Verification items for the finished model (mm, model axes). A direction names the side the tool comes from. Coordinates: 2 decimals unless noted, no trailing zeros. Order: outer loops, then holes, each group sorted by start corner. A loop starts at its lowest first (then second) coordinate and runs counter-clockwise, first axis right, second up.
Q1. Depth check by flat-ended pin: P1, Ø3, axis at x = 2.5, z = 6.5, coming from the +Y side; P2, Ø2, axis at x = 24, y = 18.5, coming from the +Z side; P3, Ø3, axis at x = 29.5, z = 4, coming from the -Y side; P4, Ø1.8, axis at y = 10.5, z = 4.5, coming from the +X side. Enter the tip coordinate at first touch or a pass-through.
Q2. Cross-section at C-C, the plane z = 6.5. Record the boundary of the cut face in (x, y), and give its area (3 significant figures).
Q3. Thickness scan on line 1 (Y direction, x = 36.2, z = 1.5); line 2 (X direction, y = 12.25, z = 6.75); line 3 (X direction, y = 12, z = 1.5). Record the ranges inside material, lowest first.
Q4. Draft check along X on faces 1 (the cylindrical face through (34.7, 13.06, 1.01)), 2 (the flat face through (40, 8, 1)), 3 (the flat face through (27.119, 17.922, 6.028)), 4 (the flat face through (28, 13, 8)). Enter one of: pulls with the +X half, pulls with the -X half, needs draft (parallel to the pull), parting line crosses it, or undercut.
Q5. Cross-section at B-B, the plane y = 15. Record the boundary of the cut face in (x, z).
Q6. Set-up check for faces 5 (the flat face through (33.2, 13, 5)), 6 (the flat face through (0, 8, 4)), 7 (the flat face through (5, 14.5, 5)), 8 (the flat face through (10, 8, 5)): record each of +Z, -Z, +X, -X, +Y, -Y from which the full face is reachable in a straight line by a thin tool's end or side.
Q7. Cross-section at D-D, the plane x = 6. Record the boundary of the cut face in (y, z), and give its area (3 significant figures).
Q8. Cross-section at A-A, the plane x = 36.2. Record the boundary of the cut face in (y, z).
from build123d import *

# Parameters (mm, degrees)
F0_W     = 40
F0_H     = 16
F1_DEPTH = 2
F2_W     = 10
F2_H     = 13
F2_W_2   = 13
F2_H_2   = 6
F3_DEPTH = 6
F4_R     = 1.5
F5_DEPTH = 25
F7_DEPTH = 4


with BuildPart() as f1:
    # F0 (on Top) → F1 (new body)
    with BuildSketch(Plane.XY):
        with Locations((20, 8)):
            Rectangle(F0_W, F0_H)
    extrude(amount=F1_DEPTH)

    # F2 (on face) → F3 (join)
    with BuildSketch(Plane.XY.offset(2)):
        with Locations((5, 8)):
            Rectangle(F2_W, F2_H)
        with Locations((26.7, 13)):
            Rectangle(F2_W_2, F2_H_2)
    extrude(amount=F3_DEPTH)

    # F4 (on face) → F5 (cut)
    with BuildSketch(Plane.XY.offset(2)):
        with Locations((17.2, 12.58387)):
            Circle(F4_R)
        with Locations((36.2, 12.996209)):
            Circle(F4_R)
    extrude(amount=-F5_DEPTH, mode=Mode.SUBTRACT)

    # F6 (on face) → F7 (join)
    with BuildSketch(Plane.XY.offset(8)):
        with BuildLine():
            Line((33.196565, 19.791735), (20.869566, 16))
            Line((20.869566, 16), (21.372473, 16))
            Line((21.372473, 16), (33.448326, 19.669136))
            ThreePointArc((33.448326, 19.669136), (34.091376, 20.578656), (34.9574, 19.878127))
            Line((34.9574, 19.878127), (35.180375, 19.999125))
            ThreePointArc((35.180375, 19.999125), (34.092116, 20.817116), (33.196565, 19.791735))
        make_face()
    extrude(amount=-F7_DEPTH)


solid = f1.part
Check values:
1. P1: stops at y = 14.5
1. P2: passes through
1. P3: stops at y = 10
1. P4: stops at x = 33.2
2. outline: (0, 1.5) - (10, 1.5) - (10, 14.5) - (0, 14.5) - close; (20.2, 10) - (33.2, 10) - (33.2, 16) - (21.37, 16) - (33.45, 19.67) arc R0.76 cw (long way) to (34.96, 19.88) - (35.18, 20) arc R1 ccw to (33.2, 19.79) - (20.87, 16) - (20.2, 16) - close
2. area: 211 mm2
3. line 1: y = 0 to 11.5, 14.5 to 16
3. line 2: x = 0 to 10, 20.2 to 33.2
3. line 3: x = 0 to 15.82, 18.58 to 35.08, 37.32 to 40
4. face 1: undercut
4. face 2: pulls with the +X half
4. face 3: pulls with the -X half
4. face 4: needs draft
5. outline: (0, 0) - (40, 0) - (40, 2) - (33.2, 2) - (33.2, 8) - (20.2, 8) - (20.2, 2) - (0, 2) - close
6. face 5: +Z, +X, -Y
6. face 6: +Z, -Z, -X, +Y, -Y
6. face 7: +Z, -X, +Y
6. face 8: +Z, +Y, -Y
7. outline: (0, 0) - (16, 0) - (16, 2) - (14.5, 2) - (14.5, 8) - (1.5, 8) - (1.5, 2) - (0, 2) - close
7. area: 110 mm2
8. outline: (0, 0) - (11.5, 0) - (11.5, 2) - (0, 2) - close; (14.5, 0) - (16, 0) - (16, 2) - (14.5, 2) - close
